from build123d import *

# Parameters (mm, degrees)
BOSS_EXTRUDE1_DEPTH = 5
BOSS_EXTRUDE1_TAPER = 20
BOSS_EXTRUDE2_DEPTH = 2
CUT_EXTRUDE1_START  = -1
CUT_EXTRUDE1_DEPTH  = 1
CHAMFER1_SIZE       = 1
CUT_EXTRUDE2_REACH  = 16.357
SKETCH4_R           = 3.5
FILLET1_R           = 1


with BuildPart() as part:
    # Sketch1 → Boss-Extrude1 (new body)
    with BuildSketch(Plane(origin=(0, 0, 0), x_dir=(1, 0, 0), z_dir=(0, 1, 0))):
        with BuildLine():
            ThreePointArc((-5.75, 9.75), (-8.578427125, 8.578427125), (-9.75, 5.75))
            Line((-9.75, 5.75), (-9.75, -5.75))
            ThreePointArc((-9.75, -5.75), (-8.578427125, -8.578427125), (-5.75, -9.75))
            Line((-5.75, -9.75), (5.75, -9.75))
            ThreePointArc((5.75, -9.75), (8.578427125, -8.578427125), (9.75, -5.75))
            Line((9.75, -5.75), (9.75, 5.75))
            ThreePointArc((9.75, 5.75), (8.578427125, 8.578427125), (5.75, 9.75))
            Line((5.75, 9.75), (-5.75, 9.75))
        make_face()
    extrude(amount=BOSS_EXTRUDE1_DEPTH, taper=BOSS_EXTRUDE1_TAPER)

    # Sketch2 → Boss-Extrude2 (add)
    with BuildSketch(Plane.XZ):
        with BuildLine():
            Line((-5.75, 7.5), (5.75, 7.5))
            ThreePointArc((5.75, 7.5), (6.987436867, 6.987436867), (7.5, 5.75))
            Line((7.5, 5.75), (7.5, -5.75))
            ThreePointArc((7.5, -5.75), (6.987436867, -6.987436867), (5.75, -7.5))
            Line((5.75, -7.5), (-5.75, -7.5))
            ThreePointArc((-5.75, -7.5), (-6.987436867, -6.987436867), (-7.5, -5.75))
            Line((-7.5, -5.75), (-7.5, 5.75))
            ThreePointArc((-7.5, 5.75), (-6.987436867, 6.987436867), (-5.75, 7.5))
        make_face()
        with BuildLine():
            Line((-5.5, 6.5), (5.5, 6.5))
            ThreePointArc((5.5, 6.5), (6.207106781, 6.207106781), (6.5, 5.5))
            Line((6.5, 5.5), (6.5, -5.5))
            ThreePointArc((6.5, -5.5), (6.207106781, -6.207106781), (5.5, -6.5))
            Line((5.5, -6.5), (-5.5, -6.5))
            ThreePointArc((-5.5, -6.5), (-6.207106781, -6.207106781), (-6.5, -5.5))
            Line((-6.5, -5.5), (-6.5, 5.5))
            ThreePointArc((-6.5, 5.5), (-6.207106781, 6.207106781), (-5.5, 6.5))
        make_face(mode=Mode.SUBTRACT)
    extrude(amount=BOSS_EXTRUDE2_DEPTH)

    # Sketch3 → Cut-Extrude1 (cut)
    with BuildSketch(Plane.XZ.offset(CUT_EXTRUDE1_START)):
        with BuildLine():
            Line((5.5, 6.5), (-5.5, 6.5))
            ThreePointArc((-5.5, 6.5), (-6.207106781, 6.207106781), (-6.5, 5.5))
            Line((-6.5, 5.5), (-6.5, -5.5))
            ThreePointArc((-6.5, -5.5), (-6.207106781, -6.207106781), (-5.5, -6.5))
            Line((-5.5, -6.5), (5.5, -6.5))
            ThreePointArc((5.5, -6.5), (6.207106781, -6.207106781), (6.5, -5.5))
            Line((6.5, -5.5), (6.5, 5.5))
            ThreePointArc((6.5, 5.5), (6.207106781, 6.207106781), (5.5, 6.5))
        make_face()
    extrude(amount=CUT_EXTRUDE1_DEPTH, mode=Mode.SUBTRACT)

    # Chamfer1
    chamfer1_edges = [part.edges().sort_by_distance(p)[0] for p in [
        (6.207106781, 1, 6.207106781),
        (6.5, 1, 0),
        (6.207106781, 1, -6.207106781),
        (0, 1, -6.5),
        (-6.207106781, 1, -6.207106781),
        (-6.5, 1, 0),
        (-6.207106781, 1, 6.207106781),
        (0, 1, 6.5),
    ]]
    chamfer(chamfer1_edges, length=CHAMFER1_SIZE - 0.0001)  # a hair under: the kernel refuses the full size

    # Sketch4 → Cut-Extrude2 (cut, up to next)
    with BuildSketch(Plane.XZ.offset(-1), mode=Mode.PRIVATE) as cut_extrude2_sk1:
        with Locations(Location((0, 0, 0), (0, 0, 270))):
            Circle(SKETCH4_R)
    cut_extrude2_tool1 = extrude(cut_extrude2_sk1.sketch, amount=-CUT_EXTRUDE2_REACH, mode=Mode.PRIVATE) & part.part
    add(cut_extrude2_tool1.solids().sort_by_distance((0, 1, 0))[0], mode=Mode.SUBTRACT)

    # Fillet1
    fillet1_edges = [part.edges().sort_by_distance(p)[0] for p in [
        (7.291598021, 5, 7.291598021),
        (7.930148829, 5, 0),
        (7.291598021, 5, -7.291598021),
        (0, 5, -7.930148829),
        (-7.291598021, 5, -7.291598021),
        (-7.930148829, 5, 0),
        (-7.291598021, 5, 7.291598021),
        (0, 5, 7.930148829),
    ]]
    fillet(fillet1_edges, radius=FILLET1_R)


solid = part.part
Source: CAD feature listing. Evaluate the final solid. Frame: model axes, mm. A direction names the side the tool comes from. Coordinates: 2 decimals unless noted, no trailing zeros. Loops run counter-clockwise (first coordinate to the right, second up) from the corner with the lowest first, then second, coordinate; pieces in that order, holes last. Notation, with made-up numbers: (7.5, 68.5) - (52.5, 68.5) arc R24 cw to (52.5, 101.5) - close; hole circle Ø11 at (87, -6.75). An arc over 180 degrees is marked (long way). One line per item, written item: value. Start each with the question number.
1. Mould query, pull axis X, two halves, no side actions, for faces 5 (the flat face through (0, -1, -7.5)), 6 (the flat face through (-6, 0.5, 0.1)), 7 (the cylindrical face through (-6.199, -0.986, -6.215)), 8 (the cylindrical face through (-7.001, -0.986, 6.974)). Classes: pulls with the +X half, pulls with the -X half, needs draft (parallel to the pull), parting line crosses it, or undercut.
2. Set-up query: faces 1 (the flat face through (-7.5, -1, 0)), 2 (the cylindrical face through (7.001, -0.986, -6.974)), 3 (the flat face through (0, -1, 7.5)), 4 (the flat face through (0, -1, -6.5)). Return all of +Z, -Z, +X, -X, +Y, -Y with unobstructed straight access to the full face (end or side cutting, diameter ignored); none if empty.
3. Contact query for flat-ended pins moving along their axis: P1, Ø1.6, axis at y = -0.5, z = -1.5, coming from the -X side; P2, Ø0.6, axis at x = 1.5, y = -1.5, coming from the +Z side; P3, Ø0.6, axis at x = 1.5, y = -1, coming from the -Z side. Output: stop coordinate, or through.
4. Ray query, L1, parallel to Z at x = 4.75, y = -1.5; L2, parallel to Y at x = -4.5, z = 2.5; L3, parallel to X at y = 0.5, z = 3. Return the intervals inside material, ascending.
5. Section A-A (y = -0.25). Return the cut outline in (x, z), and give its area (3 significant figures).
Verdict:
1. face 5: needs draft
1. face 6: undercut
1. face 7: undercut
1. face 8: pulls with the -X half
2. face 1: +Z, -Z, -X, -Y
2. face 2: -Z, +X, -Y
2. face 3: +Z, +X, -X, -Y
2. face 4: -Y
3. P1: stops at x = -9.75
3. P2: stops at z = 7.5
3. P3: stops at z = -7.5
4. L1: z = -7.5 to -6.5, 6.5 to 7.5
4. L2: y = 1 to 5
4. L3: x = -9.57 to -6, 6 to 9.57
5. outline: (-7.5, -5.75) arc R1.75 ccw to (-5.75, -7.5) - (5.75, -7.5) arc R1.75 ccw to (7.5, -5.75) - (7.5, 5.75) arc R1.75 ccw to (5.75, 7.5) - (-5.75, 7.5) arc R1.75 ccw to (-7.5, 5.75) - close; hole (-6.5, -5.5) arc R1 ccw to (-5.5, -6.5) - (5.5, -6.5) arc R1 ccw to (6.5, -5.5) - (6.5, 5.5) arc R1 ccw to (5.5, 6.5) - (-5.5, 6.5) arc R1 ccw to (-6.5, 5.5) - close
5. area: 54.2 mm2
